from build123d import *

# Parameters (mm, degrees)
SKETCH1_R           = 11
SKETCH1_R_2         = 9
BOSS_EXTRUDE1_DEPTH = 8
BOSS_EXTRUDE2_DEPTH = 2


with BuildPart() as part:
    # Sketch1 → Boss-Extrude1 (new body)
    with BuildSketch(Plane.XY):
        Circle(SKETCH1_R)
        Circle(SKETCH1_R_2, mode=Mode.SUBTRACT)
    extrude(amount=BOSS_EXTRUDE1_DEPTH)

    # Sketch2 → Boss-Extrude2 (add, symmetric)
    with BuildSketch(Plane(origin=(0, 0, 0), x_dir=(1, 0, 0), z_dir=(0, 1, 0))):
        Polygon((-11, 0), (-11, 6), (-9.8, 6), (-8, 4.2), (-9, 4.2), (-9, 0), align=None)
        Polygon((9, 0), (11, 0), (11, 6), (9.8, 6), (8, 4.2), (9, 4.2), align=None)
    extrude(amount=BOSS_EXTRUDE2_DEPTH, both=True)


solid = part.part
Work out the finished part from the listing and answer in its coordinate system (mm). A direction names the side the tool comes from. Coordinates: 2 decimals unless noted, no trailing zeros. Order: outer loops, then holes, each group sorted by start corner. A loop starts at its lowest first (then second) coordinate and runs counter-clockwise, first axis right, second up. Notation, with made-up numbers: (34.5, 72) - (70.5, 72) arc R30 ccw to (70.5, 102) - close; hole circle Ø3 at (5.5, 74.25). An arc over 180 degrees is marked (long way). Put each result on its own line as item: value. Start each with the question number.
1) Flat-ended cylindrical pins translate along their axes: pin 1 (1.5 mm diameter, centred on x = 1, z = 2.5, fed in from +Y); pin 2 (1.5 mm diameter, centred on x = 1, y = 8.5, fed in from -Z); pin 3 (0.5 mm diameter, centred on x = -8.5, y = 0, fed in from +Z). Find the tip coordinate at first contact, or state that the pin passes through.
2) For a pull along X with two mould halves and no side action, classify faces 4 (the cylindrical face through (-2.38, -10.74, 3.94)), 5 (the flat face through (9, 0, -2)), 6 (the flat face through (10, 2, -3)) as released by +X, released by -X, zero draft, split by the parting line, or undercut.
3) For faces 1 (the flat face through (-9, 0, -2)), 2 (the flat face through (10, -2, -3)), 3 (the flat face through (8.9, 0, -5.1)), determine the directions among +Z, -Z, +X, -X, +Y, -Y from which every point of the face is accessible in a straight line to the end or side of a thin tool.
4) Find the intervals of material crossed by line 1 (Y direction, x = 0, z = 3.5); line 2 (Z direction, x = 7.25, y = 7); line 3 (X direction, y = 1.25, z = 7), in increasing order. Write a range as from..to.
5) Find section C-C (y = 1). Give the vertices of the cut face in (x, z).
6) Find section A-A (z = -3.5). Give the vertices of the cut face in (x, y).
7) Find section D-D (z = 0.5). Give the vertices of the cut face in (x, y), plus the area to 3 significant figures.
8) Find section B-B (x = 0). Give the vertices of the cut face in (y, z).
Results list:
1. pin 1: stops at y = 11
1. pin 2: stops at z = 0
1. pin 3: stops at z = -4.2
2. face 4: split by the parting line
2. face 5: undercut
2. face 6: zero draft
3. face 1: +Y, -Y
3. face 2: -Z, +X, -X, -Y
3. face 3: -Z, +Y, -Y
4. line 1: y = -11..-9, 9..11
4. line 2: z = 0..8
4. line 3: x = -10.93..-8.91, 8.91..10.93
5. outline: (-11, -6) - (-9.8, -6) - (-8, -4.2) - (-9, -4.2) - (-9, 0) - (-8.94, 0) - (-8.94, 8) - (-10.95, 8) - (-10.95, 0) - (-11, 0) - close; (8, -4.2) - (9.8, -6) - (11, -6) - (11, 0) - (10.95, 0) - (10.95, 8) - (8.94, 8) - (8.94, 0) - (9, 0) - (9, -4.2) - close
6. outline: (-11, -2) - (-9, -2) - (-9, 2) - (-11, 2) - close; (9, -2) - (11, -2) - (11, 2) - (9, 2) - close
7. outline: circle Ø22 at (0, 0); hole circle Ø18 at (0, 0)
7. area: 126 mm^2
8. outline: (-11, 0) - (-9, 0) - (-9, 8) - (-11, 8) - close; (9, 0) - (11, 0) - (11, 8) - (9, 8) - close
